Part model, mm, in its own coordinate system. A direction names the side the tool comes from. Round coordinates to 2 decimals unless told otherwise and drop trailing zeros. Loops run counter-clockwise (first coordinate to the right, second up) from the corner with the lowest first, then second, coordinate; pieces in that order, holes last. Notation, with made-up numbers: (45.5, -17) -> (59.5, -17) arc R21 ccw to (59.5, 5) -> close; hole circle Ø4 at (60, -32.5). An arc over 180 degrees is marked (long way). Use a Markdown table: item, result. Add a question column.
Item 1: Which spindle directions (+Z, -Z, +X, -X, +Y, -Y) get a long thin tool onto all of the face, cutting with end or side? Do faces 4 (the face through (6, 3.1, 13)), 5 (the face through (0, 8.4, 1.8)), 6 (the face through (6, 17.85, 7)). Say none if no direction does.
Item 2: Two-plate mould, pull along Y, no slides. Class faces 1 (the face through (7, 10, 0)), 2 (the face through (6, 17, 11.8)), 3 (the face through (7.2, 19.3, 13.23)): pulls with the +Y half, pulls with the -Y half, needs draft (parallel to the pull), parting line crosses it, or undercut.
Item 3: Cut at B-B, the plane z = 11. List the corners of the cut face in (x, y).
Item 4: Cut at C-C, the plane x = 1.5. List the corners of the cut face in (y, z).
Item 5: Probe line 1 (Y direction, x = 1.75, z = 7.75); line 2 (Z direction, x = 6.75, y = 13); line 3 (X direction, y = 5.5, z = 11). List the from-to ranges inside material, lowest first. Write a range as [from, to].
Item 6: Flat gauge pins, fed straight in: pin 1 (1.6 mm diameter, centred on x = 4, z = 13, fed in from +Y); pin 2 (3.5 mm diameter, centred on y = 12.5, z = 6.5, fed in from -X); pin 3 (1.5 mm diameter, centred on x = 4, y = 6.5, fed in from +Z). Where does each tip first touch, or does it go through?
Item 7: Cut at A-A, the plane y = 8.15. List the corners of the cut face in (x, z).
```python
from build123d import *

# Parameters (mm, degrees)
F0_W     = 14.2
F0_H     = 19.9
F1_DEPTH = 13.8
F2_DEPTH = 12
F4_DEPTH = 12.2
F6_DEPTH = 2.001
F7_ANGLE = 180
F8_R     = 2


with BuildPart() as f1:
    # F0 (on Top) → F1 (new body)
    with BuildSketch(Plane.XY):
        with Locations((7.1, 9.95)):
            Rectangle(F0_W, F0_H)
    extrude(amount=F1_DEPTH)

    # F0 (on Top) → F2 (join)
    with BuildSketch(Plane.XY):
        with Locations((7.1, 9.95)):
            Rectangle(F0_W, F0_H)
    extrude(amount=F2_DEPTH)

    # F3 (on face) → F4 (cut)
    with BuildSketch(Plane(origin=(0, 0, 0), x_dir=(0, -1, 0), z_dir=(-1, 0, 0))):
        Polygon((-3.1, 13.8), (-16.8, 13.8), (-16.8, 11.8), (-17.85, 11.8), (-17.85, 2), (-2.05, 2), (-2.05, 11.8), (-3.1, 11.8), align=None)
    extrude(amount=-F4_DEPTH, mode=Mode.SUBTRACT)

    # F5 (on face) → F6 (cut, through all)
    with BuildSketch(Plane(origin=(12.2, 0, 0), x_dir=(0, -1, 0), z_dir=(-1, 0, 0))):
        with BuildLine():
            ThreePointArc((-11.9975769926, 8.4152777778), (-11.75, 8.2), (-11.5024230074, 8.4152777778))
            ThreePointArc((-11.5024230074, 8.4152777778), (-11.75, 8.45), (-11.9975769926, 8.4152777778))
        make_face()
        with BuildLine():
            ThreePointArc((-11.9975769926, 8.4152777778), (-11.75, 8.45), (-11.5024230074, 8.4152777778))
            ThreePointArc((-11.5024230074, 8.4152777778), (-11.5006064875, 8.4325966693), (-11.5, 8.45))
            ThreePointArc((-11.5, 8.45), (-11.7674033307, 8.6993935125), (-11.9975769926, 8.4152777778))
        make_face()
        with BuildLine():
            ThreePointArc((-8.3975769926, 8.4152777778), (-8.15, 8.2), (-7.9024230074, 8.4152777778))
            ThreePointArc((-7.9024230074, 8.4152777778), (-8.15, 8.45), (-8.3975769926, 8.4152777778))
        make_face()
        with BuildLine():
            ThreePointArc((-8.3975769926, 8.4152777778), (-8.15, 8.45), (-7.9024230074, 8.4152777778))
            ThreePointArc((-7.9024230074, 8.4152777778), (-7.9006064875, 8.4325966693), (-7.9, 8.45))
            ThreePointArc((-7.9, 8.45), (-8.1674033307, 8.6993935125), (-8.3975769926, 8.4152777778))
        make_face()
        with BuildLine():
            ThreePointArc((-8.3975769926, 6.6847222222), (-8.15, 6.65), (-7.9024230074, 6.6847222222))
            ThreePointArc((-7.9024230074, 6.6847222222), (-8.15, 6.9), (-8.3975769926, 6.6847222222))
        make_face()
        with BuildLine():
            ThreePointArc((-7.9, 6.65), (-7.9006064875, 6.6674033307), (-7.9024230074, 6.6847222222))
            ThreePointArc((-7.9024230074, 6.6847222222), (-8.15, 6.65), (-8.3975769926, 6.6847222222))
            ThreePointArc((-8.3975769926, 6.6847222222), (-8.1674033307, 6.4006064875), (-7.9, 6.65))
        make_face()
        with BuildLine():
            ThreePointArc((-11.9975769926, 6.6847222222), (-11.75, 6.65), (-11.5024230074, 6.6847222222))
            ThreePointArc((-11.5024230074, 6.6847222222), (-11.75, 6.9), (-11.9975769926, 6.6847222222))
        make_face()
        with BuildLine():
            ThreePointArc((-11.5, 6.65), (-11.5006064875, 6.6674033307), (-11.5024230074, 6.6847222222))
            ThreePointArc((-11.5024230074, 6.6847222222), (-11.75, 6.65), (-11.9975769926, 6.6847222222))
            ThreePointArc((-11.9975769926, 6.6847222222), (-11.7674033307, 6.4006064875), (-11.5, 6.65))
        make_face()
    extrude(amount=-F6_DEPTH, mode=Mode.SUBTRACT)

    # F5 (on face) → F7 (revolve)
    with BuildSketch(Plane(origin=(12.2, 0, 0), x_dir=(0, -1, 0), z_dir=(-1, 0, 0))):
        with BuildLine():
            Line((-12.65, 7.55), (-10.85, 7.55))
            ThreePointArc((-10.85, 7.55), (-11.0313835191, 8.0918397856), (-11.5024230074, 8.4152777778))
            ThreePointArc((-11.5024230074, 8.4152777778), (-11.75, 8.2), (-11.9975769926, 8.4152777778))
            ThreePointArc((-11.9975769926, 8.4152777778), (-12.4686164809, 8.0918397856), (-12.65, 7.55))
        make_face()
        with BuildLine():
            Line((-9.05, 7.55), (-7.25, 7.55))
            ThreePointArc((-7.25, 7.55), (-7.4313835191, 8.0918397856), (-7.9024230074, 8.4152777778))
            ThreePointArc((-7.9024230074, 8.4152777778), (-8.15, 8.2), (-8.3975769926, 8.4152777778))
            ThreePointArc((-8.3975769926, 8.4152777778), (-8.8686164809, 8.0918397856), (-9.05, 7.55))
        make_face()
    revolve(axis=Axis((12.2, 11.75, 7.55), (0, -1, 0)), revolution_arc=F7_ANGLE)

    # F8
    f8_edges = [f1.edges().sort_by_distance(p)[0] for p in [
        (7.1, 0, 0),
        (7.1, 19.9, 0),
        (7.1, 19.9, 13.8),
        (7.1, 0, 13.8),
        (14.2, 0, 6.9),
        (14.2, 19.9, 6.9),
    ]]
    fillet(f8_edges, radius=F8_R)


solid = f1.part
```
A:
| question | item | result |
|---|---|---|
| 1 | face 4 | +Z, -X |
| 1 | face 5 | +Z, -Z, -X, +Y, -Y |
| 1 | face 6 | -X |
| 2 | face 1 | needs draft |
| 2 | face 2 | undercut |
| 2 | face 3 | pulls with the +Y half |
| 3 | outline | (0, 0) -> (12.2, 0) arc R2 ccw to (14.2, 2) -> (14.2, 17.9) arc R2 ccw to (12.2, 19.9) -> (0, 19.9) -> (0, 17.85) -> (12.2, 17.85) -> (12.2, 2.05) -> (0, 2.05) -> close |
| 4 | outline | (0, 2) arc R2 ccw to (2, 0) -> (17.9, 0) arc R2 ccw to (19.9, 2) -> (19.9, 11.8) arc R2 ccw to (17.9, 13.8) -> (16.8, 13.8) -> (16.8, 11.8) -> (17.85, 11.8) -> (17.85, 2) -> (2.05, 2) -> (2.05, 11.8) -> (3.1, 11.8) -> (3.1, 13.8) -> (2, 13.8) arc R2 ccw to (0, 11.8) -> close |
| 5 | line 1 | y = [0, 2.05], [17.85, 19.9] |
| 5 | line 2 | z = [0, 2] |
| 5 | line 3 | x = [12.2, 14.2] |
| 6 | pin 1 | stops at y = 19.86 |
| 6 | pin 2 | stops at x = 11.33 |
| 6 | pin 3 | stops at z = 2 |
| 7 | outline | (0, 0) -> (14.2, 0) -> (14.2, 6.4) -> (12.2, 6.4) -> (12.2, 2) -> (0, 2) -> close; (12.2, 6.9) -> (14.2, 6.9) -> (14.2, 8.2) -> (12.2, 8.2) arc R0.65 ccw to start; (12.2, 8.7) -> (14.2, 8.7) -> (14.2, 13.8) -> (12.2, 13.8) -> close |
